Geometry: final body of the model. Coordinates: model frame, mm. Face numbers are marked on the shaded views. Give positions to 0.01 mm unless a question says otherwise; leave off trailing zeros. Write each loop counter-clockwise with the first axis right and the second up, starting at its lowest first coordinate (ties: lowest second). Pieces come first, ordered by that corner, then holes. Notation, with made-up numbers: (21, 58) -> (55, 58) arc R27 cw to (55, 77) -> close; hole circle Ø9 at (-28.75, 59). An arc over 180 degrees is marked (long way). Answer in a Markdown table with one row per item. Add a question column.
Item 1: First-contact query: P1, Ø3.5, axis at y = 9.5, z = -1, coming from the -X side; P2, Ø4.5, axis at y = -5.33, z = 14.23, coming from the +X side; P3, Ø4.5, axis at x = -13.66, y = 7.51, coming from the +Z side; P4, Ø3, axis at y = 0.5, z = 9.5, coming from the +X side. Flat tips, straight axial feed; report the tip coordinate or a pass-through.
Item 2: Material intervals for probe 1 along X at (y, z) = (13.5, 17.5); probe 2 along X at (y, z) = (-8.5, 14.75); probe 3 along Z at (x, y) = (-1.5, 6), sorted ascending. Write a range as from..to.
Item 3: Section query A-A on z = 8.25. Output: boundary loops of the cut face in (x, y), plus the area to 3 significant figures.
Item 4: Draft query along X for the marked faces 1, 2 and 3. Return one class per face: +X half, -X half, draft (parallel to the pull), parting line (faces both ways), or undercut.
Item 5: Section query C-C on x = 19. Output: boundary loops of the cut face in (y, z).
Item 6: Section query D-D on x = 8.5. Output: boundary loops of the cut face in (y, z).
Item 7: Section query B-B on x = -8.5. Output: boundary loops of the cut face in (y, z).
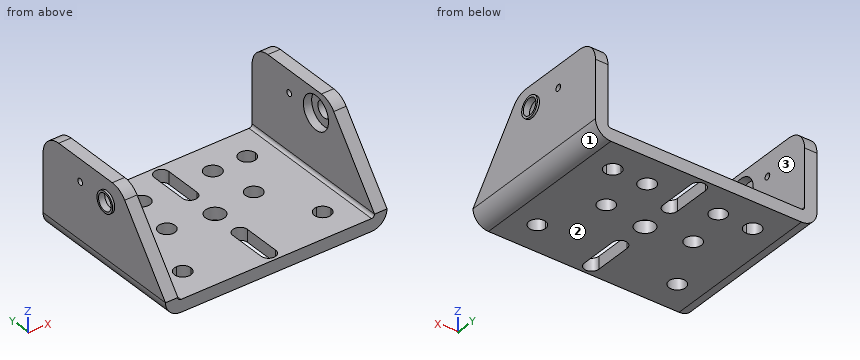
```python
from build123d import *

# Parameters (mm, degrees)
ESBO_O1_W                        = 47.5
ESBO_O1_H                        = 39
FLANGE_BASE1_DEPTH               = 3
ESBO_O6_R                        = 2.3
CORTE_EXTRUS_O1_DEPTH            = 10
ARESTA_FLANGE1_STRIP_W           = 13.4732
ARESTA_FLANGE1_STRIP_H           = 3
ARESTA_FLANGE1_STRIP_CUT_DEPTH   = 39
ARESTA_FLANGE1_STRIP_2_W         = 13.4732
ARESTA_FLANGE1_STRIP_2_H         = 3
ARESTA_FLANGE1_STRIP_CUT_2_DEPTH = 39
ARESTA_FLANGE1_DEPTH             = 39
ARESTA_FLANGE1_BEND_DEPTH        = 39
ESBO_O13_R                       = 2
ESBO_O13_R_2                     = 0.75
CORTE_EXTRUS_O2_DEPTH            = 70
FILETE1_R                        = 5
ESBO_O14_R                       = 1.997873176
ESBO_O14_R_2                     = 2.026064888
ESBO_O14_R_3                     = 2
CORTE_EXTRUS_O4_DEPTH            = 3
BOSS_EXTRUDE1_START              = 0.5
SKETCH1_R                        = 2.5
SKETCH1_R_2                      = 2
BOSS_EXTRUDE1_DEPTH              = 0.5
SKETCH2_R                        = 4
CUT_EXTRUDE8_DEPTH               = 2


# Sheet-metal steps are written as plain solids
with BuildPart() as part:
    # Esboço1 → Flange-base1 (new body)
    with BuildSketch(Plane.XY):
        with Locations((3.243735783, -4.490936556)):
            Rectangle(ESBO_O1_W, ESBO_O1_H)
    extrude(amount=-FLANGE_BASE1_DEPTH)

    # Esboço6 → Corte-extrusão1 (cut)
    with BuildSketch(Plane.XY):
        with BuildLine():
            Line((-13.656264217, 5.509063444), (-13.656264217, 7.509063444))
            Line((-13.656264217, 7.509063444), (-11.656264217, 7.509063444))
            ThreePointArc((-11.656264217, 7.509063444), (-15.070477779, 8.923277006), (-13.656264217, 5.509063444))
        make_face()
        with BuildLine():
            Line((-11.656264217, 7.509063444), (-13.656264217, 7.509063444))
            Line((-13.656264217, 7.509063444), (-13.656264217, 5.509063444))
            ThreePointArc((-13.656264217, 5.509063444), (-12.242050654, 6.094849882), (-11.656264217, 7.509063444))
        make_face()
        with BuildLine():
            ThreePointArc((-11.656264217, -16.490936556), (-12.242050654, -15.076722994), (-13.656264217, -14.490936556))
            Line((-13.656264217, -14.490936556), (-13.656264217, -16.490936556))
            Line((-13.656264217, -16.490936556), (-11.656264217, -16.490936556))
        make_face()
        with BuildLine():
            Line((-13.656264217, -16.490936556), (-13.656264217, -14.490936556))
            ThreePointArc((-13.656264217, -14.490936556), (-15.070477779, -17.905150118), (-11.656264217, -16.490936556))
            Line((-11.656264217, -16.490936556), (-13.656264217, -16.490936556))
        make_face()
        with Locations((3.243735783, -4.490936556)):
            Circle(ESBO_O6_R)
        with BuildLine():
            Line((4.993735783, 7.509063444), (1.493735783, 7.509063444))
            Line((1.493735783, 7.509063444), (1.493735783, 3.523823043))
            ThreePointArc((1.493735783, 3.523823043), (3.243735783, 1.773823043), (4.993735783, 3.523823043))
            Line((4.993735783, 3.523823043), (4.993735783, 7.509063444))
        make_face()
        with BuildLine():
            Line((1.493735783, 12.523823043), (1.493735783, 7.509063444))
            Line((1.493735783, 7.509063444), (4.993735783, 7.509063444))
            Line((4.993735783, 7.509063444), (4.993735783, 12.523823043))
            ThreePointArc((4.993735783, 12.523823043), (3.243735783, 14.273823043), (1.493735783, 12.523823043))
        make_face()
        with BuildLine():
            Line((1.493735783, -12.505696155), (1.493735783, -16.490936556))
            Line((1.493735783, -16.490936556), (4.993735783, -16.490936556))
            Line((4.993735783, -16.490936556), (4.993735783, -12.505696155))
            ThreePointArc((4.993735783, -12.505696155), (3.243735783, -10.755696155), (1.493735783, -12.505696155))
        make_face()
        with BuildLine():
            Line((4.993735783, -16.490936556), (1.493735783, -16.490936556))
            Line((1.493735783, -16.490936556), (1.493735783, -21.505696155))
            ThreePointArc((1.493735783, -21.505696155), (3.243735783, -23.255696155), (4.993735783, -21.505696155))
            Line((4.993735783, -21.505696155), (4.993735783, -16.490936556))
        make_face()
        with BuildLine():
            ThreePointArc((22.143735783, -16.490936556), (21.557949346, -15.076722994), (20.143735783, -14.490936556))
            Line((20.143735783, -14.490936556), (20.143735783, -16.490936556))
            Line((20.143735783, -16.490936556), (18.143735783, -16.490936556))
            ThreePointArc((18.143735783, -16.490936556), (20.143735783, -18.490936556), (22.143735783, -16.490936556))
        make_face()
        with BuildLine():
            Line((20.143735783, -16.490936556), (20.143735783, -14.490936556))
            ThreePointArc((20.143735783, -14.490936556), (18.729522221, -15.076722994), (18.143735783, -16.490936556))
            Line((18.143735783, -16.490936556), (20.143735783, -16.490936556))
        make_face()
        with BuildLine():
            ThreePointArc((22.143735783, 7.509063444), (20.143735783, 9.509063444), (18.143735783, 7.509063444))
            Line((18.143735783, 7.509063444), (20.143735783, 7.509063444))
            Line((20.143735783, 7.509063444), (20.143735783, 5.509063444))
            ThreePointArc((20.143735783, 5.509063444), (21.557949346, 6.094849882), (22.143735783, 7.509063444))
        make_face()
        with BuildLine():
            Line((20.143735783, 7.509063444), (18.143735783, 7.509063444))
            ThreePointArc((18.143735783, 7.509063444), (18.729522221, 6.094849882), (20.143735783, 5.509063444))
            Line((20.143735783, 5.509063444), (20.143735783, 7.509063444))
        make_face()
    extrude(amount=-CORTE_EXTRUS_O1_DEPTH, mode=Mode.SUBTRACT)

    # Aresta-Flange1 strip (across the edge) → Aresta-Flange1 strip cut (cut)
    with BuildSketch(Plane(origin=(26.993735783, -23.990936556, 0), x_dir=(-1, 0, 0), z_dir=(0, 1, 0))):
        with Locations((-6, -1.5)):
            Rectangle(ARESTA_FLANGE1_STRIP_W, ARESTA_FLANGE1_STRIP_H)
    extrude(amount=ARESTA_FLANGE1_STRIP_CUT_DEPTH, mode=Mode.SUBTRACT)

    # Aresta-Flange1 strip 2 (across the edge) → Aresta-Flange1 strip cut 2 (cut)
    with BuildSketch(Plane(origin=(-20.506264217, 15.009063444, 0), x_dir=(1, 0, 0), z_dir=(0, -1, 0))):
        with Locations((-6, -1.5)):
            Rectangle(ARESTA_FLANGE1_STRIP_2_W, ARESTA_FLANGE1_STRIP_2_H)
    extrude(amount=ARESTA_FLANGE1_STRIP_CUT_2_DEPTH, mode=Mode.SUBTRACT)

    # Aresta-Flange1 section (across the edge) → Aresta-Flange1 (add)
    with BuildSketch(Plane(origin=(26.993735783, -23.990936556, 0), x_dir=(-1, 0, 0), z_dir=(0, 1, 0))):
        with BuildLine():
            Line((-3, 0.7366), (-3, 19.5))
            Line((-3, 19.5), (0, 19.5))
            Line((0, 19.5), (0, 0.7366))
            ThreePointArc((0, 0.7366), (0.215745145, 0.215745145), (0.7366, 0))
            Line((0.7366, 0), (0.7366, -3))
            ThreePointArc((0.7366, -3), (-1.905575199, -1.905575199), (-3, 0.7366))
        make_face()
    extrude(amount=ARESTA_FLANGE1_DEPTH)

    # Aresta-Flange1 section 2 (across the edge) → Aresta-Flange1 bend (add)
    with BuildSketch(Plane(origin=(-20.506264217, 15.009063444, 0), x_dir=(1, 0, 0), z_dir=(0, -1, 0))):
        with BuildLine():
            Line((-3, 0.7366), (-3, 19.5))
            Line((-3, 19.5), (0, 19.5))
            Line((0, 19.5), (0, 0.7366))
            ThreePointArc((0, 0.7366), (0.215745145, 0.215745145), (0.7366, 0))
            Line((0.7366, 0), (0.7366, -3))
            ThreePointArc((0.7366, -3), (-1.905575199, -1.905575199), (-3, 0.7366))
        make_face()
    extrude(amount=ARESTA_FLANGE1_BEND_DEPTH)

    # Esboço13 → Corte-extrusão2 (cut)
    with BuildSketch(Plane.ZY.offset(23.506264217)):
        with Locations((14.234737, -5.325205188)):
            Circle(ESBO_O13_R)
        with Locations((14.234737, 3.174794812)):
            Circle(ESBO_O13_R_2)
        Polygon((0.7366, -23.990936556), (19.5, -23.990936556), (19.5, -9.490936556), align=None)
    extrude(amount=-CORTE_EXTRUS_O2_DEPTH, mode=Mode.SUBTRACT)

    # Filete1
    filete1_edges = [part.edges().sort_by_distance(p)[0] for p in [
        (28.493735783, 15.009063444, 19.5),
        (-22.006264217, 15.009063444, 19.5),
        (-22.006264217, -9.490936556, 19.5),
        (28.493735783, -9.490936556, 19.5),
    ]]
    fillet(filete1_edges, radius=FILETE1_R)

    # Esboço14 → Corte-extrusão4 (cut)
    with BuildSketch(Plane.XY):
        with Locations((-5.331264217, 7.509063444)):
            Circle(ESBO_O14_R)
        with Locations((11.818735783, 7.509063444)):
            Circle(ESBO_O14_R_2)
        with Locations((13.743735783, -2.990936556)):
            Circle(ESBO_O14_R_3)
        with Locations(Location((-7.256264217, -2.990936556, 0), (0, 0, 180))):
            Circle(ESBO_O14_R_3)
    extrude(amount=-CORTE_EXTRUS_O4_DEPTH, mode=Mode.SUBTRACT)

    # Sketch1 → Boss-Extrude1 (add)
    with BuildSketch(Plane.ZY.offset(23.506264217).offset(BOSS_EXTRUDE1_START)):
        with Locations(Location((14.234737, -5.325205188, 0), (0, 0, 180))):
            Circle(SKETCH1_R)
        with Locations((14.234737, -5.325205188)):
            Circle(SKETCH1_R_2, mode=Mode.SUBTRACT)
    boss_extrude1 = extrude(amount=-BOSS_EXTRUDE1_DEPTH)

    # Sketch2 → Cut-Extrude8 (cut)
    with BuildSketch(Plane(origin=(-20.506264217, 0, 0), x_dir=(0, 0, -1), z_dir=(1, 0, 0))):
        with Locations((-14.234737, -5.325205188)):
            Circle(SKETCH2_R)
    cut_extrude8 = extrude(amount=-CUT_EXTRUDE8_DEPTH, mode=Mode.SUBTRACT)

    # Mirror1: Boss-Extrude1, Cut-Extrude8 across plane
    add(boss_extrude1.mirror(Plane.ZY.offset(-3.243735783)))
    add(cut_extrude8.mirror(Plane.ZY.offset(-3.243735783)), mode=Mode.SUBTRACT)


solid = part.part
```
Findings below:
| question | item | result |
|---|---|---|
| 1 | P1 | stops at x = -23.51 |
| 1 | P2 | stops at x = 30.49 |
| 1 | P3 | stops at z = 0 |
| 1 | P4 | stops at x = 29.99 |
| 2 | probe 1 | x = -23.51..-20.51, 26.99..29.99 |
| 2 | probe 2 | x = -23.51..-22.51, 28.99..29.99 |
| 2 | probe 3 | z = -3..0 |
| 3 | outline | (-23.51, -18.18) -> (-20.51, -18.18) -> (-20.51, 15.01) -> (-23.51, 15.01) -> close; (26.99, -18.18) -> (29.99, -18.18) -> (29.99, 15.01) -> (26.99, 15.01) -> close |
| 3 | area | 199 mm^2 |
| 4 | face 1 | +X half |
| 4 | face 2 | draft |
| 4 | face 3 | undercut |
| 5 | outline | (-23.99, -3) -> (-18.13, -3) -> (-18.13, 0) -> (-23.99, 0) -> close; (-14.85, -3) -> (5.87, -3) -> (5.87, 0) -> (-14.85, 0) -> close; (9.15, -3) -> (15.01, -3) -> (15.01, 0) -> (9.15, 0) -> close |
| 6 | outline | (-23.99, -3) -> (15.01, -3) -> (15.01, 0) -> (-23.99, 0) -> close |
| 7 | outline | (-23.99, -3) -> (-4.56, -3) -> (-4.56, 0) -> (-23.99, 0) -> close; (-1.42, -3) -> (15.01, -3) -> (15.01, 0) -> (-1.42, 0) -> close |
